Design review of the part built by this model. Coordinates are the model's own, in mm. A direction names the side the tool comes from. Coordinates: 2 decimals unless noted, no trailing zeros. Loops run counter-clockwise (first coordinate to the right, second up) from the corner with the lowest first, then second, coordinate; pieces in that order, holes last. Notation, with made-up numbers: (21, -3.5) -> (76, -3.5) arc R10 ccw to (76, 11.5) -> close; hole circle Ø8 at (85, -32.75). An arc over 180 degrees is marked (long way). One line per item, written item: value. Start each with the question number.
1. Add section C-C on z = -2.5. Write out the cut boundary in (x, y).
2. Add section A-A on x = 0. Write out the cut boundary in (y, z).
3. Add section D-D on y = -5.75. Write out the cut boundary in (x, z).
4. Draft analysis for pull direction Y (two halves, no side actions). For faces 4 (the cylindrical face through (0, -2, -8)), 5 (the flat face through (4, -4, -2)), 6 (the cylindrical face through (1.172, 8.923, -3.972)), state which applies: pulls with the +Y half, pulls with the -Y half, needs draft (parallel to the pull), parting line crosses it, or undercut.
5. Add section B-B on y = 0. Write out the cut boundary in (x, z), plus the area to 3 significant figures.
6. Machinability: for faces 1 (the cylindrical face through (7.8, 0, -4)), 2 (the cylindrical face through (-1.86, 2.92, -10.83)), 3 (the cylindrical face through (-0.59, 4.46, -1.09)), which of the approach directions +Z, -Z, +X, -X, +Y, -Y give a long, thin tool a straight path to every point of the face, cutting with its end or side? Answer none if there is none.
7. For probe 1 along Y at (x, z) = (-3.5, -4.05); probe 2 along Y at (x, z) = (0, -7); probe 3 along Z at (x, y) = (-3.75, 4), list the stretches that pass through material, from the lowest coordinate up.
8. Insertion check: pin 1 (9 mm diameter, centred on x = -4, y = -4, fed in from -Z); pin 2 (2 mm diameter, centred on x = 7, y = 0, fed in from -Z); pin 3 (2 mm diameter, centred on y = 2.5, z = -7.5, fed in from -X); pin 4 (1 mm diameter, centred on y = 4.5, z = -13, fed in from +X). Each pin has a flat end and moves straight along its axis. Give the tip position at first contact, or say it passes through.
```python
from build123d import *

# Parameters (mm, degrees)
SKETCH1_R             = 4.5
BOSS_EXTRUDE1_DEPTH   = 2
SKETCH2_R             = 9
BOSS_EXTRUDE2_DEPTH   = 4
SKETCH3_R             = 3.463787736
BOSS_EXTRUDE3_DEPTH   = 10
M2X0_4_TAPPED_HOLE1_D = 1.6
SKETCH7_R             = 2
CUT_EXTRUDE3_DEPTH    = 17
CHAMFER1_SIZE         = 0.2


with BuildPart() as part:
    # Sketch1 → Boss-Extrude1 (new body)
    with BuildSketch(Plane.XY):
        Circle(SKETCH1_R)
    extrude(amount=-BOSS_EXTRUDE1_DEPTH)

    # Sketch2 → Boss-Extrude2 (add)
    with BuildSketch(Plane(origin=(0, 0, -2), x_dir=(-1, 0, 0), z_dir=(0, 0, -1))):
        Circle(SKETCH2_R)
    extrude(amount=BOSS_EXTRUDE2_DEPTH)

    # Sketch3 → Boss-Extrude3 (add)
    with BuildSketch(Plane(origin=(0, 0, -6), x_dir=(-1, 0, 0), z_dir=(0, 0, -1))):
        Circle(SKETCH3_R)
    extrude(amount=BOSS_EXTRUDE3_DEPTH)

    # M2x0.4 Tapped Hole1 (through all)
    with Locations(Plane.XY.offset(-2)):
        with Locations((-3.5, 6.062177826), (-3.5, -6.062177826), (7, 0)):
            Hole(M2X0_4_TAPPED_HOLE1_D / 2)

    # Sketch7 → Cut-Extrude3 (cut, through all)
    with BuildSketch(Plane.XY):
        Circle(SKETCH7_R)
    extrude(amount=-CUT_EXTRUDE3_DEPTH, mode=Mode.SUBTRACT)

    # Chamfer1
    chamfer1_edges = [part.edges().sort_by_distance(p)[0] for p in [
        (3.463787736, 0, -16),
        (-4.5, 0, 0),
        (-2, 0, -16),
        (-2, 0, 0),
    ]]
    chamfer(chamfer1_edges, length=CHAMFER1_SIZE)


solid = part.part
```
Worked answers:
1. outline: circle Ø18 at (0, 0); hole circle Ø1.6 at (-3.5, -6.06); hole circle Ø1.6 at (-3.5, 6.06); hole circle Ø4 at (0, 0); hole circle Ø1.6 at (7, 0)
2. outline: (-9, -6) -> (-3.46, -6) -> (-3.46, -15.8) -> (-3.26, -16) -> (-2.2, -16) -> (-2, -15.8) -> (-2, -0.2) -> (-2.2, 0) -> (-4.3, 0) -> (-4.5, -0.2) -> (-4.5, -2) -> (-9, -2) -> close; (2, -15.8) -> (2.2, -16) -> (3.26, -16) -> (3.46, -15.8) -> (3.46, -6) -> (9, -6) -> (9, -2) -> (4.5, -2) -> (4.5, -0.2) -> (4.3, 0) -> (2.2, 0) -> (2, -0.2) -> close
3. outline: (-6.92, -6) -> (-4.24, -6) -> (-4.24, -2) -> (-6.92, -2) -> close; (-2.76, -6) -> (6.92, -6) -> (6.92, -2) -> (-2.76, -2) -> close
4. face 4: undercut
4. face 5: needs draft
4. face 6: parting line crosses it
5. outline: (-9, -6) -> (-3.46, -6) -> (-3.46, -15.8) -> (-3.26, -16) -> (-2.2, -16) -> (-2, -15.8) -> (-2, -0.2) -> (-2.2, 0) -> (-4.3, 0) -> (-4.5, -0.2) -> (-4.5, -2) -> (-9, -2) -> close; (2, -15.8) -> (2.2, -16) -> (3.26, -16) -> (3.46, -15.8) -> (3.46, -6) -> (6.2, -6) -> (6.2, -2) -> (4.5, -2) -> (4.5, -0.2) -> (4.3, 0) -> (2.2, 0) -> (2, -0.2) -> close; (7.8, -6) -> (9, -6) -> (9, -2) -> (7.8, -2) -> close
5. area: 88.7 mm²
6. face 1: +Z, -Z
6. face 2: -Z
6. face 3: +Z
7. probe 1: y = -8.29 to -6.86, -5.26 to 5.26, 6.86 to 8.29
7. probe 2: y = -3.46 to -2, 2 to 3.46
7. probe 3: z = -6 to -2
8. pin 1: stops at z = -16
8. pin 2: stops at z = -6
8. pin 3: stops at x = -3.12
8. pin 4: passes through
